```python
from build123d import *

# Parameters (mm, degrees)
F1_DEPTH = 20
F2_DEPTH = 10


# Not quite as in the source:
# - a feature names something its author has since deleted; it is built from what else it names


with BuildPart() as f1:
    # F0 (on Top) → F1 (new body)
    with BuildSketch(Plane.XY):
        Polygon((-50, 21), (-50, 0), (-48, 0), (0, 0), (0, 1.5), (-48.5, 1.5), (-48.5, 19.5), (0, 19.5), (0, 21), align=None)
    extrude(amount=F1_DEPTH)

    # F0 (on Top) → F2 (join)
    with BuildSketch(Plane.XY):
        with BuildLine():
            ThreePointArc((-50, 0), (-62.5, -12.5), (-75, 0))
            Line((-75, 0), (-77, 0))
            ThreePointArc((-77, 0), (-62.5, -14.5), (-48, 0))
            Line((-48, 0), (-50, 0))
        make_face()
    extrude(amount=F2_DEPTH)


solid = f1.part
```
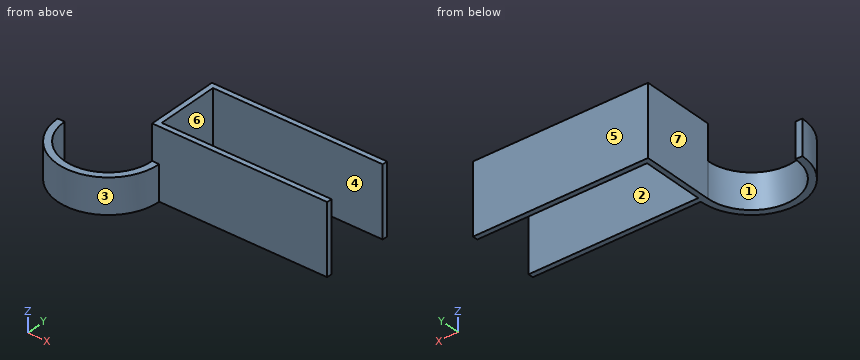
For this review, take the finished solid that the model builds, in its own axes (mm). Face numbers are marked on the shaded views. A direction names the side the tool comes from. Round coordinates to 2 decimals unless told otherwise and drop trailing zeros. Write each loop counter-clockwise with the first axis right and the second up, starting at its lowest first coordinate (ties: lowest second). Pieces come first, ordered by that corner, then holes.
1) Insertion check: pin 1 Ø10 at (y, z) = (9.5, 8) entering from -X; pin 2 Ø5 at (x, z) = (-19, 11) entering from -Y; pin 3 Ø5 at (x, z) = (-63, 3) entering from -Y; pin 4 Ø1.6 at (x, z) = (-76, 5.5) entering from +Y. Each pin has a flat end and moves straight along its axis. Give the tip position at first contact, or say it passes through.
Answer below:
pin 1: stops at x = -50
pin 2: stops at y = 0
pin 3: stops at y = -14.5
pin 4: stops at y = 0
2) Take a section at C-C on z = 14.25. Give the boundary of the cut face in (x, y).
Answer below:
outline: (-50, 0) - (0, 0) - (0, 1.5) - (-48.5, 1.5) - (-48.5, 19.5) - (0, 19.5) - (0, 21) - (-50, 21) - close
3) For line 1 along Y through (x, z) = (-24, 8.5); line 2 along X through (y, z) = (11.5, 18.5); line 3 along Y through (x, z) = (-62, 2.5), list the stretches that pass through material, from the lowest coordinate up.
Answer below:
line 1: y = 0 to 1.5, 19.5 to 21
line 2: x = -50 to -48.5
line 3: y = -14.49 to -12.49
4) Take a section at A-A on x = -10. Give the boundary of the cut face in (y, z), then the cut area to 3 significant figures.
Answer below:
outline: (0, 0) - (1.5, 0) - (1.5, 20) - (0, 20) - close; (19.5, 0) - (21, 0) - (21, 20) - (19.5, 20) - close
area: 60.0 mm2
5) Machinability: for the marked faces 5, 6 and 7, which of the approach directions +Z, -Z, +X, -X, +Y, -Y give a long, thin tool a straight path to every point of the face, cutting with its end or side? Answer none if there is none.
Answer below:
face 5: +Z, -Z, +X, -X, +Y
face 6: +Z, -Z, +X
face 7: +Z, -Z, -X, +Y
6) Take a section at B-B on y = -9. Give the boundary of the cut face in (x, z), then the cut area to 3 significant figures.
Answer below:
outline: (-73.87, 0) - (-71.17, 0) - (-71.17, 10) - (-73.87, 10) - close; (-53.83, 0) - (-51.13, 0) - (-51.13, 10) - (-53.83, 10) - close
area: 53.9 mm2
7) Take a section at D-D on x = -62.5. Give the boundary of the cut face in (y, z).
Answer below:
outline: (-14.5, 0) - (-12.5, 0) - (-12.5, 10) - (-14.5, 10) - close
8) Mouldability with a two-part tool opening along Y and no side actions: class the marked faces 1, 2, 3 and 4 as +Y half, -Y half, draft (parallel to the pull), parting line (faces both ways), or undercut.
Answer below:
face 1: +Y half
face 2: undercut
face 3: -Y half
face 4: undercut
